Check sheet for the modelled part. Datum: model origin and axes. Units: mm. A direction names the side the tool comes from. Give positions to 0.01 mm unless a question says otherwise; leave off trailing zeros. Loops run counter-clockwise (first coordinate to the right, second up) from the corner with the lowest first, then second, coordinate; pieces in that order, holes last. Notation, with made-up numbers: (30.25, -18.75) -> (65.25, -18.75) arc R18 ccw to (65.25, 14.25) -> close; hole circle Ø3 at (4.5, 78). An arc over 180 degrees is marked (long way). Answer as CSV lines item,"result". Start each with the question number.
(1) Material ranges on line 1 (Z direction, x = 23.5, y = -30); line 2 (Z direction, x = 2.75, y = 0); line 3 (Z direction, x = 11.25, y = -5.5), recorded low to high. Write a range as from..to.
(2) Section check B-B on y = -22.5. Enter the section's corners in (x, z), plus the area to 3 significant figures.
(3) Gauge pin test, flat ends, axial feed: pin 1 Ø10 at (x, y) = (13, 13) entering from +Z; pin 2 Ø1 at (x, z) = (9, -7) entering from -Y; pin 3 Ø4 at (y, z) = (-8.5, -18.5) entering from +X; pin 4 Ø22.5 at (y, z) = (0, 0) entering from -X. Record the tip position at first contact, or that the pin passes through.
(4) Section check C-C on x = 6. Enter the section's corners in (y, z), plus the area to 3 significant figures.
(5) Section check A-A on z = 0. Enter the section's corners in (x, y), plus the area to 3 significant figures.
(6) Release check for a two-part mould opening along Z. For faces 4 (the face through (12.325, -45.693, 25.14)), 5 (the face through (12.32, -19.4, 12.64)), 6 (the face through (12.32, 34.99, 0.77)) record: pulls with the +Z half, pulls with the -Z half, needs draft (parallel to the pull), parting line crosses it, or undercut.
(7) Section check D-D on z = -24. Enter the section's corners in (x, y).
(8) Access from +Z, -Z, +X, -X, +Y, -Y to the whole of each face (thin tool, end or side, straight path). Record for faces 1 (the face through (17.4, -43.4, 25.11)), 2 (the face through (12.325, -45.693, -25.14)), 3 (the face through (12, -37, -15)).
Autodesk Inventor part; units mm, degrees
ref_plane "YZ Plane" through (0, 0, 0) normal (1, 0, 0) x (0, 1, 0)
ref_plane "XZ Plane" through (0, 0, 0) normal (0, 1, 0) x (-1, 0, 0)
ref_plane "XY Plane" through (0, 0, 0) normal (0, 0, 1) x (1, 0, 0)
sketch "Sketch1" plane through (0, 0, 0) normal (1, 0, 0) x (0, 1, 0)
  arc A0 (0, -35) -> (0, 35) centre (0, 0) ccw
  circle A1 centre (0, 0) radius 20
  circle A2 centre (0, 0) radius 14
  line L0 (0, 35) -> (-40, 35)
  line L1 (-40, 35) -> (-51.547, 15)
  line L2 (-40, 35) -> (-40, 2.9908) construction
  line L3 (-51.547, 15) -> (-21.547, 15)
  line L4 (-21.547, 15) -> (-17.1937, 10.2166)
  line L5 (0, 0) -> (45.2071, 0) construction
  arc A3 (-15.748, -29) -> (0, 33) centre (0, 0) ccw
  line L6 (0, 33) -> (-38.8453, 33)
  line L7 (-38.8453, 33) -> (-48.0829, 17)
  line L8 (-48.0829, 17) -> (-15.152, 17)
  line L9 (-15.152, 17) -> (-13.1879, 15.0359)
  line L10 (-15.152, 17) -> (-12.3744, 17) construction
  line L11 (0, -35) -> (-40, -35)
  line L12 (-40, -35) -> (-51.547, -15)
  line L13 (-40, -35) -> (-40, -2.9908) construction
  line L14 (-51.547, -15) -> (-21.547, -15)
  line L15 (-21.547, -15) -> (-17.1937, -10.2166)
  line L16 (0, -33) -> (-38.8453, -33)
  line L17 (-38.8453, -33) -> (-48.0829, -17)
  line L18 (-48.0829, -17) -> (-15.152, -17)
  line L19 (-15.152, -17) -> (-13.1879, -15.0359)
  point P0 (0, -33)
  point P1 (-13.1879, -15.0359)
  point P2 (-17.1937, -10.2166)
  dimension "d0" = 70
  dimension "d9" = 15
  dimension "d17" = 6
  dimension "d32" = 40
  dimension "d43" = 20
  dimension "d44" = 30
  dimension "d45" = 30
  dimension "d47" = 2
  dimension "d48" = 45
  dimension "d49" = 132.305
  dimension "d50" = 1.3067
  dimension "d51" = 30.6595
  dimension "d52" = 29
  dimension "d54" = 2.9907
extrude "Extrusion3" add sketch "Sketch1" along normal blind 25 contours L11 L12 L14 L15 A1 L19 L18 L17 L16 A3 L6 L7 L8 L9 L4 L3 L1 L0 A0
extrude "Extrusion4" add sketch "Sketch1" along normal blind 10 contours A1 | A1 L9 L8 L7 L6 A3 L16 L17 L18 L19
sketch "Sketch2" plane through (0, 0, 0) normal (-1, 0, 0) x (0, 0, 1)
  line L0 (-15, -21.547) -> (-15, -51.547)
  line L1 (-10.2166, -17.1937) -> (-15, -21.547)
  line L2 (-15, -21.547) -> (-10.2166, -17.1937)
  arc A0 (-10.2166, -17.1937) -> (10.2166, -17.1937) centre (0, 0) ccw
  arc A1 (-10.2166, -17.1937) -> (10.2166, -17.1937) centre (0, 0) ccw
  line L3 (15, -51.547) -> (15, -21.547)
  line L4 (15, -21.547) -> (10.2166, -17.1937)
  line L5 (15, -21.547) -> (10.2166, -17.1937)
properties part number "Brazo_3DPrint"
Working result:
1,line 1,"z = -35..-33, -17..-15, 15..17, 33..35"
1,line 2,"z = -35..-14, 14..35"
1,line 3,"z = -35..-33, 33..35"
2,outline,"(0, -35) -> (25, -35) -> (25, -33) -> (10, -33) -> (10, -17) -> (25, -17) -> (25, -15) -> (0, -15) -> close; (0, 15) -> (25, 15) -> (25, 17) -> (10, 17) -> (10, 33) -> (25, 33) -> (25, 35) -> (0, 35) -> close"
2,area,"520 mm^2"
3,pin 1,"stops at z = 34.07"
3,pin 2,"stops at y = -18.91"
3,pin 3,"stops at x = 10"
3,pin 4,"passes through"
4,outline,"(-51.55, -15) -> (-40, -35) -> (0, -35) arc R35 ccw to (0, 35) -> (-40, 35) -> (-51.55, 15) -> (-21.55, 15) -> (-17.19, 10.22) arc R20 ccw to (-17.19, -10.22) -> (-21.55, -15) -> close; hole circle Ø28 at (0, 0)"
4,area,"3,710 mm^2"
5,outline,"(0, -20) -> (10, -20) -> (10, -14) -> (0, -14) -> close; (0, 14) -> (10, 14) -> (10, 33) -> (25, 33) -> (25, 35) -> (0, 35) -> close"
5,area,"300 mm^2"
6,face 4,"pulls with the +Z half"
6,face 5,"undercut"
6,face 6,"parting line crosses it"
7,outline,"(0, -46.35) -> (25, -46.35) -> (25, -44.04) -> (10, -44.04) -> (10, 22.65) -> (25, 22.65) -> (25, 25.48) -> (0, 25.48) -> close"
8,face 1,"+X"
8,face 2,"-Z, +X, -X, -Y"
8,face 3,"+X, -X, -Y"
